Print and shaded views of the part. All mm, measured from the part's lowest x, y and z. A direction names the side the tool comes from. Round coordinates to 2 decimals unless told otherwise and drop trailing zeros. Loops run counter-clockwise (first coordinate to the right, second up) from the corner with the lowest first, then second, coordinate; pieces in that order, holes last. Notation, with made-up numbers: (41.25, 27.25) -> (59.25, 27.25) arc R6 cw to (59.25, 32.25) -> close; hole circle Ø1 at (-13.75, -0.75). An arc over 180 degrees is marked (long way). Answer as CSV lines item,"result".
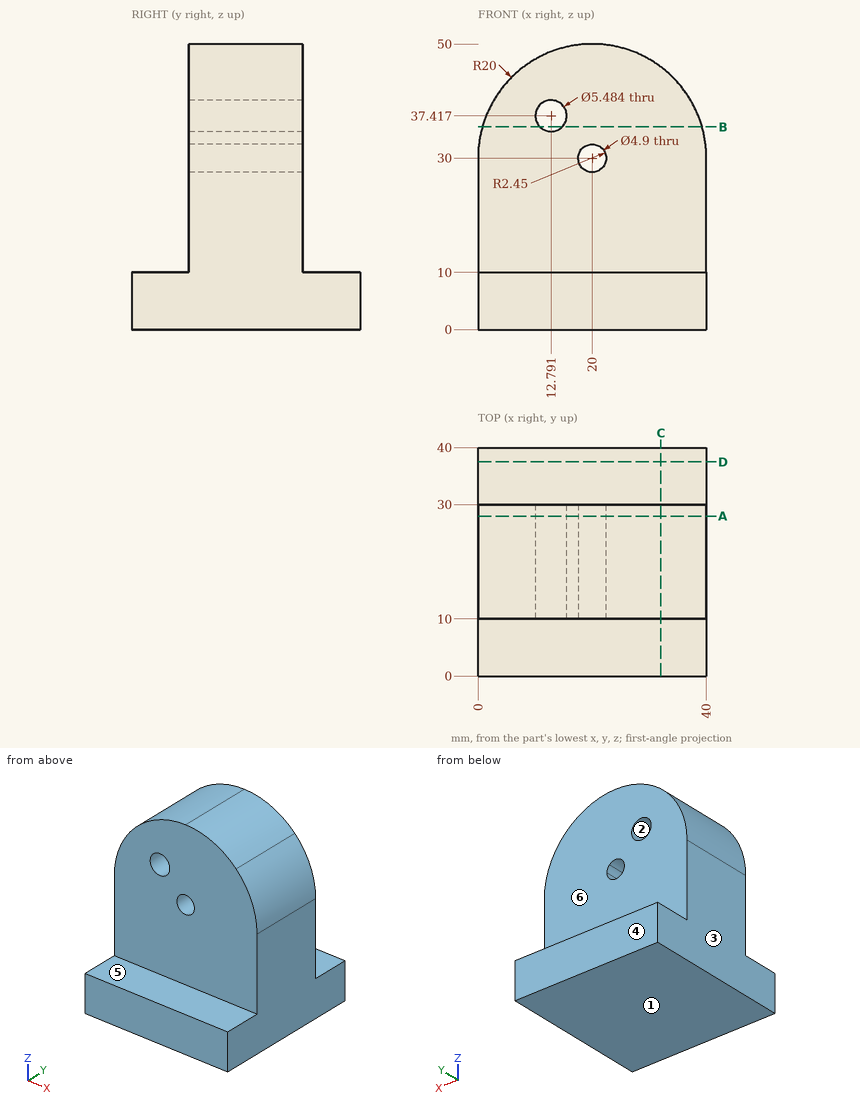
Q1. Tool access for the marked faces 4, 5 and 6: list every direction of +Z, -Z, +X, -X, +Y, -Y with a clear straight run to the whole face (end or side of a thin tool).
Results:
face 4,"+Z, -Z, +X, -X, +Y"
face 5,"+Z, +X, -X, -Y"
face 6,"+Z, +X, -X, +Y"
Q2. Two-plate mould, pull along X, no slides. Class the marked faces 1, 2 and 3: pulls with the +X half, pulls with the -X half, needs draft (parallel to the pull), parting line crosses it, or undercut.
Results:
face 1,"needs draft"
face 2,"undercut"
face 3,"pulls with the -X half"
Q3. Probe L1, parallel to X at y = 20, z = 30; L2, parallel to Z at x = 37.5, y = 9; L3, parallel to Y at x = 5, z = 29. List the from-to ranges inside material, lowest first. Write a range as [from, to].
Results:
L1,"[0, 17.55], [22.45, 40]"
L2,"[0, 10]"
L3,"[10, 30]"
Q4. Slice it at A-A, the plane y = 28. Count the separate pieces of the cut face and the enclosed holes in it, and give its area (3 significant figures).
Results:
separate pieces,"1"
enclosed holes,"2"
area,"1,790 mm2"
Q5. Drop flat-ended pins along their axis: pin 1 Ø20 at (x, z) = (28.5, 32.5) entering from +Y; pin 2 Ø11 at (x, y) = (19.5, 4) entering from +Z; pin 3 Ø3 at (x, y) = (32, 13) entering from +Z. Give the stop position or say it passes through.
Results:
pin 1,"y = 30"
pin 2,"z = 10"
pin 3,"z = 47.02"
Q6. Slice it at B-B, the plane z = 35.5. Give the cut face in (x, y), and give its area (3 significant figures).
Results:
outline,"(0.77, 10) -> (10.83, 10) -> (10.83, 30) -> (0.77, 30) -> close; (14.75, 10) -> (39.23, 10) -> (39.23, 30) -> (14.75, 30) -> close"
area,"691 mm2"
Q7. Slice it at D-D, the plane y = 37.5. Give the cut face in (x, z), and give its area (3 significant figures).
Results:
outline,"(0, 0) -> (40, 0) -> (40, 10) -> (0, 10) -> close"
area,"400 mm2"
Q8. Slice it at C-C, the plane x = 32. Give the cut face in (y, z), and give its area (3 significant figures).
Results:
outline,"(0, 0) -> (40, 0) -> (40, 10) -> (30, 10) -> (30, 46) -> (10, 46) -> (10, 10) -> (0, 10) -> close"
area,"1,120 mm2"
